Autodesk Inventor part; units mm, degrees
ref_plane "YZ Plane" through (0, 0, 0) normal (1, 0, 0) x (0, 1, 0)
ref_plane "XZ Plane" through (0, 0, 0) normal (0, 1, 0) x (-1, 0, 0)
ref_plane "XY Plane" through (0, 0, 0) normal (0, 0, 1) x (1, 0, 0)
sketch "Sketch1" plane through (0, 0, 0) normal (0, 0, 1) x (1, 0, 0)
  circle A0 centre (0, 0) radius 19.5
  circle A1 centre (15, 0) radius 2.5
  circle A2 centre (-7.5, 12.9904) radius 2.5
  circle A3 centre (-7.5, -12.9904) radius 2.5
  dimension "d0" = 39
  dimension "d1" = 5
  dimension "d2" = 15
  dimension "d5" = 360
extrude "Extrusion1" add sketch "Sketch1" along normal blind 5
sketch "Sketch2" plane through (0, 0, 0) normal (0, 0, -1) x (-1, 0, 0)
  circle A0 centre (0, 0) radius 5
  dimension "d9" = 10
extrude "Extrusion2" cut sketch "Sketch2" against normal blind 4
fillet "Fillet1" radius 2 1 edges at (-19.5, 0, 5)
properties part number "AA049" material "ABS Plastic"
Work out the finished part from the listing and answer in its coordinate system (mm). A direction names the side the tool comes from. Give positions to 0.01 mm unless a question says otherwise; leave off trailing zeros. Order: outer loops, then holes, each group sorted by start corner. A loop starts at its lowest first (then second) coordinate and runs counter-clockwise, first axis right, second up.
1. Straight lines are drawn through the part: L1, parallel to X at y = -2, z = 3.25; L2, parallel to Z at x = 4, y = -1; L3, parallel to Y at x = -7.5, z = 3.5. For each, find the intervals that lie inside material, in ascending order.
Result sheet:
L1: x = -19.38 to -4.58, 4.58 to 13.5, 16.5 to 19.38
L2: z = 4 to 5
L3: y = -17.93 to -15.49, -10.49 to 10.49, 15.49 to 17.93
2. For faces 4 (the flat face through (0, 0, 4)), 5 (the cylindrical face through (-10, 13, 2)), determine the directions among +Z, -Z, +X, -X, +Y, -Y from which every point of the face is accessible in a straight line to the end or side of a thin tool.
Result sheet:
face 4: -Z
face 5: +Z, -Z
3. Each of these flat-tipped pins is pushed along its axis until it touches: P1, Ø1, axis at y = 14.5, z = 3.5, coming from the -X side; P2, Ø3, axis at x = 0.5, y = 2.5, coming from the -Z side. Where does it stop, or does it pass through?
Result sheet:
P1: stops at x = -13.51
P2: stops at z = 4
4. The mould has two halves that part along X. Classify faces 1 (the cylindrical face through (17.385, -0.751, 2.465)), 2 (the flat face through (0, 0, 5)), 3 (the cylindrical face through (-2.539, -19.334, 1.479)): released by +X, released by -X, zero draft, split by the parting line, or undercut.
Result sheet:
face 1: undercut
face 2: zero draft
face 3: split by the parting line
5. Section B-B, the plane z = 2.1 is taken. Determine the outline of the cut face in (x, y).
Result sheet:
outline: circle Ø39 at (0, 0); hole circle Ø5 at (-7.5, -12.99); hole circle Ø5 at (-7.5, 12.99); hole circle Ø10 at (0, 0); hole circle Ø5 at (15, 0)
6. Section A-A, the plane x = 0 is taken. Determine the outline of the cut face in (y, z).
Result sheet:
outline: (-19.5, 0) - (-5, 0) - (-5, 4) - (5, 4) - (5, 0) - (19.5, 0) - (19.5, 3) arc R2 ccw to (17.5, 5) - (-17.5, 5) arc R2 ccw to (-19.5, 3) - close
7. Section C-C, the plane x = -5.5 is taken. Give the number of separate pieces and of enclosed holes in the cut face, and give its area (3 significant figures).
Result sheet:
separate pieces: 3
enclosed holes: 0
area: 155 mm2
